Build history of the part. All positions in model axes, mm. A direction names the side the tool comes from. Give positions to 0.01 mm unless a question says otherwise; leave off trailing zeros. Order: outer loops, then holes, each group sorted by start corner. A loop starts at its lowest first (then second) coordinate and runs counter-clockwise, first axis right, second up. Notation, with made-up numbers: M 39.5,64 L 95.5,64 A25 ccw 95.5,93 Z; hole C 66.5,37.25 d6. An arc over 180 degrees is marked long. One line per item, written item: value.
from build123d import *

# Parameters (mm, degrees)
SKETCH_1_R          = 10
EXTRUDE_1_DEPTH     = 2
SKETCH_2_R          = 15.8
EXTRUDE_2_DEPTH     = 3.5
SKETCH_3_R          = 10
EXTRUDE_3_DEPTH     = 2
SKETCH_4_R          = 5
CUT_EXTRUDE_1_DEPTH = 10
CHAMFER_1_SIZE      = 0.2


with BuildPart() as part:
    # 草图1 → 凸台-拉伸1 (new body)
    with BuildSketch(Plane.XY):
        Circle(SKETCH_1_R)
    extrude(amount=EXTRUDE_1_DEPTH)

    # 草图2 → 凸台-拉伸2 (add)
    with BuildSketch(Plane.XY.offset(2)):
        Circle(SKETCH_2_R)
    extrude(amount=EXTRUDE_2_DEPTH)

    # 草图3 → 凸台-拉伸3 (add)
    with BuildSketch(Plane.XY.offset(5.5)):
        Circle(SKETCH_3_R)
    extrude(amount=EXTRUDE_3_DEPTH)

    # 草图4 → 切除-拉伸1 (cut)
    with BuildSketch(Plane.XY.offset(7.5)):
        Circle(SKETCH_4_R)
    extrude(amount=-CUT_EXTRUDE_1_DEPTH, mode=Mode.SUBTRACT)

    # 倒角1
    chamfer_1_edges = [part.edges().sort_by_distance(p)[0] for p in [
        (-15.8, 0, 2),
        (-15.8, 0, 5.5),
    ]]
    chamfer(chamfer_1_edges, length=CHAMFER_1_SIZE)


solid = part.part
1) Saw through at D-D, the plane z = 0.75. Write the cut outline in (x, y).
Check values:
outline: C 0,0 d20; hole C 0,0 d10
2) Tool access for faces 4 (the face through (-2.17, -9.76, 0.99)), 5 (the face through (-5, -2, 7.5)): list every direction of +Z, -Z, +X, -X, +Y, -Y with a clear straight run to the whole face (end or side of a thin tool).
Check values:
face 4: -Z
face 5: +Z, +X, -X, +Y, -Y
3) Mould opens along Z. For faces 1 (the face through (-2.17, -9.76, 6.49)), 2 (the face through (-0.2, -10.2, 5.5)), 3 (the face through (-5, -2, 0)) say: released by +Z, released by -Z, zero draft, split by the parting line, or undercut.
Check values:
face 1: zero draft
face 2: released by +Z
face 3: released by -Z
4) Saw through at C-C, the plane z = 4.5. Write the cut outline in (x, y), then the cut area to 3 significant figures.
Check values:
outline: C 0,0 d31.6; hole C 0,0 d10
area: 706 mm^2
5) Drill centre lines: probe 1 along Y at (x, z) = (0, 2.25); probe 2 along Z at (x, y) = (10.5, -10); probe 3 along X at (y, z) = (-2, 1.75). Where is each one in solid material? Low to high. Write a range as from..to.
Check values:
probe 1: -15.8..-5, 5..15.8
probe 2: 2..5.5
probe 3: -9.8..-4.58, 4.58..9.8
6) Pin check, flat tips, straight feed: pin 1 (1 mm diameter, centred on x = -2.5, z = 1, fed in from +Y); pin 2 (3 mm diameter, centred on y = 3, z = 5.5, fed in from -X); pin 3 (8 mm diameter, centred on x = 0, y = 0, fed in from +Z); pin 4 (1.5 mm diameter, centred on x = -12.5, z = 5.5, fed in from +Y). Stop position of each tip, or through.
Check values:
pin 1: y = 9.8
pin 2: x = -15.73
pin 3: through
pin 4: y = 10.53
7) Saw through at A-A, the plane y = 0. Write the cut outline in (x, z).
Check values:
outline: M -15.8,2.2 L -15.6,2 L -10,2 L -10,0 L -5,0 L -5,7.5 L -10,7.5 L -10,5.5 L -15.6,5.5 L -15.8,5.3 Z; M 5,0 L 10,0 L 10,2 L 15.6,2 L 15.8,2.2 L 15.8,5.3 L 15.6,5.5 L 10,5.5 L 10,7.5 L 5,7.5 Z
